from build123d import *

# Parameters (mm, degrees)
SKETCH2_W         = 22
SKETCH2_H         = 22
SWITCH_BASE_DEPTH = 12


with BuildPart() as part:
    # Sketch1 → Stick Revolve (revolve)
    with BuildSketch(Plane.XY):
        with BuildLine():
            Line((0, 0), (-11, 0))
            Line((-11, 0), (-11, 16))
            ThreePointArc((-11, 16), (-9.242640687, 20.242640687), (-5, 22))
            Line((-5, 22), (-4.5, 22))
            Line((-4.5, 22), (-4.5, 30))
            Line((-4.5, 30), (-11, 30))
            Line((-11, 30), (-11, 32))
            ThreePointArc((-11, 32), (-10.414213562, 33.414213562), (-9, 34))
            Line((-9, 34), (0, 34))
            Line((0, 34), (0, 0))
        make_face()
    revolve(axis=Axis((0, 34, 0), (0, -1, 0)))

    # Sketch2 → Switch Base (add)
    with BuildSketch(Plane.XZ):
        Rectangle(SKETCH2_W, SKETCH2_H)
    extrude(amount=-SWITCH_BASE_DEPTH)


solid = part.part
Check sheet for the modelled part. Datum: model origin and axes. Units: mm. A direction names the side the tool comes from. Round coordinates to 2 decimals unless told otherwise and drop trailing zeros. Order: outer loops, then holes, each group sorted by start corner. A loop starts at its lowest first (then second) coordinate and runs counter-clockwise, first axis right, second up.
Q1. Set-up check for faces 1 (the face through (2.38, 14.03, 10.74)), 2 (the face through (-9, 12, -8)), 3 (the face through (9, 12, -9)), 4 (the face through (0.59, 26.06, -4.46)), 5 (the face through (8, 12, 9)): record each of +Z, -Z, +X, -X, +Y, -Y from which the full face is reachable in a straight line by a thin tool's end or side.
Filled sheet:
face 1: +Y
face 2: -Z, -X, +Y
face 3: -Z, +X, +Y
face 4: none
face 5: +Z, +X, +Y
Q2. Scan lines: L1, parallel to Y at x = 4.75, z = -1; L2, parallel to Y at x = 9.25, z = 2.5; L3, parallel to Z at x = -0.25, y = 27. Record each from-to range of solid material in increasing order.
Filled sheet:
L1: y = 0 to 22, 30 to 34
L2: y = 0 to 19.87, 30 to 33.91
L3: z = -4.49 to 4.49
Q3. Cross-section at A-A, the plane y = 24. Enter the section's corners in (x, z).
Filled sheet:
outline: circle Ø9 at (0, 0)
Q4. Depth check by flat-ended pin: P1, Ø6, axis at x = -3, y = 24, coming from the +Z side; P2, Ø5, axis at x = 3.5, y = 22, coming from the +Z side; P3, Ø4, axis at y = 29.5, z = 4.5, coming from the -X side. Enter the tip coordinate at first touch or a pass-through.
Filled sheet:
P1: stops at z = 7.87
P2: stops at z = 9.4
P3: stops at x = -10.7
Q5. Draft check along Y on faces 6 (the face through (2.38, 31.01, 10.74)), 7 (the face through (0, 0, 0)), 8 (the face through (0, 30, 5)), 9 (the face through (-9, 12, 8)). Enter one of: pulls with the +Y half, pulls with the -Y half, needs draft (parallel to the pull), parting line crosses it, or undercut.
Filled sheet:
face 6: needs draft
face 7: pulls with the -Y half
face 8: undercut
face 9: pulls with the +Y half
Q6. Cross-section at B-B, the plane y = 31. Enter the section's corners in (x, z), plus the area to 3 significant figures.
Filled sheet:
outline: circle Ø22 at (0, 0)
area: 380 mm2
